For this review, use the dimensioned drawing (mm, ordinates from the lowest corner) and the shaded views. A direction names the side the tool comes from. Coordinates: 2 decimals unless noted, no trailing zeros. Write each loop counter-clockwise with the first axis right and the second up, starting at its lowest first coordinate (ties: lowest second). Pieces come first, ordered by that corner, then holes.
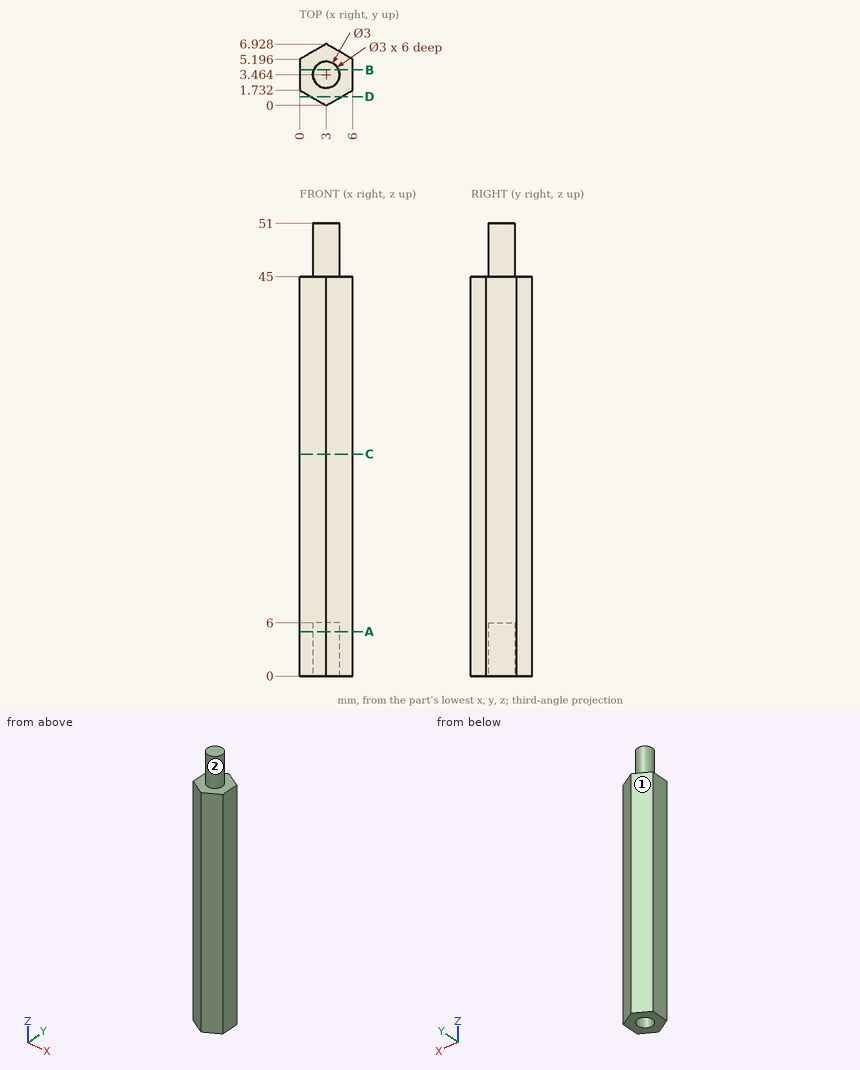
Item 1: Take a section at A-A, the plane z = 5. Write out the cut boundary in (x, y).
Solved:
outline: (0, 1.73) - (3, 0) - (6, 1.73) - (6, 5.2) - (3, 6.93) - (0, 5.2) - close; hole circle Ø3 at (3, 3.46)
Item 2: For pin 1 (3.5 mm diameter, centred on x = 3.5, y = 3, fed in from -Z); pin 2 (1 mm diameter, centred on x = 1, y = 2.5, fed in from +Z); pin 3 (2.5 mm diameter, centred on x = 3, y = 3.46, fed in from -Z), all flat-tipped, find the tip position at first contact; note any pin that passes through.
Solved:
pin 1: stops at z = 0
pin 2: stops at z = 45
pin 3: stops at z = 6
Item 3: Machinability: for the marked faces 1 and 2, which of the approach directions +Z, -Z, +X, -X, +Y, -Y give a long, thin tool a straight path to every point of the face, cutting with its end or side? Answer none if there is none.
Solved:
face 1: +Z, -Z, -X, +Y
face 2: +Z
Item 4: Take a section at B-B, the plane y = 4. Write out the cut boundary in (x, z), plus the area to 3 significant figures.
Solved:
outline: (0, 0) - (1.6, 0) - (1.6, 6) - (4.4, 6) - (4.4, 0) - (6, 0) - (6, 45) - (4.4, 45) - (4.4, 51) - (1.6, 51) - (1.6, 45) - (0, 45) - close
area: 270 mm2
Item 5: Take a section at C-C, the plane z = 25. Write out the cut boundary in (x, y), plus the area to 3 significant figures.
Solved:
outline: (0, 1.73) - (3, 0) - (6, 1.73) - (6, 5.2) - (3, 6.93) - (0, 5.2) - close
area: 31.2 mm2
Item 6: To check wall thickness, follow line 1 along Z through (x, y) = (4.5, 1); line 2 along Z through (x, y) = (1.75, 2.75); line 3 along Y through (x, z) = (2.75, 36) (1 decimal). State the ranges of each line that lie inside material, in increasing order.
Solved:
line 1: z = 0 to 45
line 2: z = 6 to 51
line 3: y = 0.1 to 6.8
Item 7: Take a section at D-D, the plane y = 1. Write out the cut boundary in (x, z), plus the area to 3 significant figures.
Solved:
outline: (1.27, 0) - (4.73, 0) - (4.73, 45) - (1.27, 45) - close
area: 156 mm2
